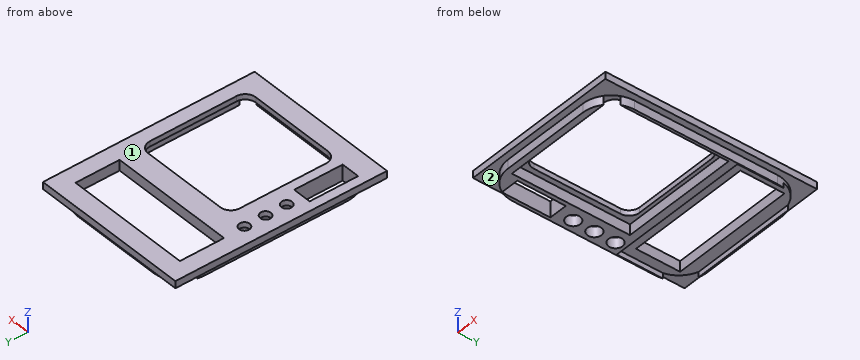
Autodesk Fusion 360 part; units mm, degrees
sketch "Skizze1" plane through (0, 0, 0) normal (0, 0, 1) x (1, 0, 0)
  line L0 (-52.263, 59.6389) -> (37.737, 59.6389)
  line L1 (37.737, 59.6389) -> (37.737, -60.3611)
  line L2 (37.737, -60.3611) -> (-52.263, -60.3611)
  line L3 (-52.263, -60.3611) -> (-52.263, 59.6389)
  dimension "d1" = 90
  dimension "d2" = 120
extrude "Extrusion1" add sketch "Skizze1" against normal blind 3
extrude "Extrusion2" add 1 faces at (-22.263, 19.6389, 0) along direction (0, 0, 1) blind 1
sketch "Skizze2" plane through (0, 0, 1) normal (0, 0, 1) x (-1, 0, 0)
  line L0 (52.263, 60.3611) -> (-37.737, 60.3611)
  line L1 (-37.737, 60.3611) -> (-37.737, -59.6389)
  line L2 (-37.737, -59.6389) -> (52.263, -59.6389)
  line L3 (52.263, -59.6389) -> (52.263, 60.3611)
  line L4 (25.263, -11.6389) -> (-23.737, -11.6389)
  line L5 (-29.737, -5.6389) -> (-29.737, 43.3611)
  line L6 (-23.737, 49.3611) -> (25.263, 49.3611)
  line L7 (31.263, 43.3611) -> (31.263, -5.6389)
  line L8 (33.263, -12.6389) -> (-31.737, -12.6389)
  line L9 (-31.737, -12.6389) -> (-31.737, 52.3611)
  line L10 (-31.737, 52.3611) -> (33.263, 52.3611)
  line L11 (33.263, 52.3611) -> (33.263, -12.6389)
  line L12 (42.763, -49.1389) -> (-28.237, -49.1389)
  line L13 (-28.237, -49.1389) -> (-28.237, -24.1389)
  line L14 (-28.237, -24.1389) -> (42.763, -24.1389)
  line L15 (42.763, -24.1389) -> (42.763, -49.1389)
  circle A0 centre (42.263, -12.1389) radius 3
  circle A1 centre (42.263, -0.1389) radius 3
  circle A2 centre (42.263, 11.8611) radius 3
  line L16 (47.013, 20.8611) -> (36.513, 20.8611)
  line L17 (36.513, 20.8611) -> (36.513, 48.3611)
  line L18 (36.513, 48.3611) -> (47.013, 48.3611)
  line L19 (47.013, 48.3611) -> (47.013, 20.8611)
  arc A3 (-29.737, -5.6389) -> (-23.737, -11.6389) centre (-23.737, -5.6389) ccw
  arc A4 (25.263, -11.6389) -> (31.263, -5.6389) centre (25.263, -5.6389) ccw
  arc A5 (31.263, 43.3611) -> (25.263, 49.3611) centre (25.263, 43.3611) ccw
  arc A6 (-23.737, 49.3611) -> (-29.737, 43.3611) centre (-23.737, 43.3611) ccw
  point P0 (31.263, -11.6389)
  point P1 (-29.737, -11.6389)
  point P2 (31.263, 49.3611)
  dimension "d7" = 61
  dimension "d8" = 61
  dimension "d10" = 11
  dimension "d11" = 65
  dimension "d12" = 65
  dimension "d13" = 8
  dimension "d19" = 25
  dimension "d20" = 71
  dimension "d23" = 8
  dimension "d24" = 6
  dimension "d25" = 6
  dimension "d26" = 9
  dimension "d28" = 6
  dimension "d29" = 6
  dimension "d30" = 12
  dimension "d31" = 9
  dimension "d32" = 9
  dimension "d33" = 12
  dimension "d34" = 10.5
  dimension "d35" = 27.5
  dimension "d36" = 12
  dimension "d37" = 5.25
  dimension "d62" = 6
  dimension "d63" = 6
  dimension "d82" = 12
sketch "Skizze3" plane through (0, 0, -3) normal (0, 0, -1) x (1, 0, 0)
  line L0 (37.737, 60.3611) -> (-52.263, 60.3611)
  line L1 (-52.263, 60.3611) -> (-52.263, -59.6389)
  line L2 (-52.263, -59.6389) -> (37.737, -59.6389)
  line L3 (37.737, -59.6389) -> (37.737, 60.3611)
  line L4 (-32.763, 56.8611) -> (18.237, 56.8611)
  line L5 (34.237, 40.8611) -> (34.237, -56.1389)
  line L6 (34.237, -56.1389) -> (-48.763, -56.1389)
  line L7 (-48.763, -56.1389) -> (-48.763, 40.8611)
  arc A0 (34.237, 40.8611) -> (18.237, 56.8611) centre (18.237, 40.8611) ccw
  arc A1 (-32.763, 56.8611) -> (-48.763, 40.8611) centre (-32.763, 40.8611) ccw
  line L8 (-52.263, 0.3611) -> (37.737, 0.3611)
  arc A2 (-48.763, -40.1389) -> (-32.763, -56.1389) centre (-32.763, -40.1389) ccw
  arc A3 (18.237, -56.1389) -> (34.237, -40.1389) centre (18.237, -40.1389) ccw
  dimension "d38" = 3.5
  dimension "d39" = 3.5
  dimension "d40" = 3.5
  dimension "d41" = 3.5
  dimension "d45" = 16
  dimension "d46" = 16
extrude "Extrusion3" add sketch "Skizze3" along normal blind 5 contours L4 L5 L7 A0 A1 L8 | L5 L6 L7 L8 A2 A3
extrude "Extrusion4" cut sketch "Skizze2" against normal blind 9 contours A1
extrude "Extrusion5" cut sketch "Skizze2" against normal blind 9 contours A0 | A2
sketch "Skizze4" plane through (0, 0, -8) normal (0, 0, -1) x (1, 0, 0)
  circle A0 centre (-42.263, -12.1389) radius 3
  circle A1 centre (-42.263, 11.8611) radius 3
  circle A2 centre (-42.263, -0.1389) radius 3
  arc A3 (-48.763, -40.1389) -> (-32.763, -56.1389) centre (-32.763, -40.1389) ccw
  line L0 (-32.763, -56.1389) -> (18.237, -56.1389)
  arc A4 (18.237, -56.1389) -> (34.237, -40.1389) centre (18.237, -40.1389) ccw
  line L1 (34.237, -40.1389) -> (34.237, 40.8611)
  arc A5 (34.237, 40.8611) -> (18.237, 56.8611) centre (18.237, 40.8611) ccw
  line L2 (18.237, 56.8611) -> (-32.763, 56.8611)
  arc A6 (-32.763, 56.8611) -> (-48.763, 40.8611) centre (-32.763, 40.8611) ccw
  line L3 (-48.763, 40.8611) -> (-48.763, -40.1389)
  circle A7 centre (-42.263, 11.8611) radius 4
  circle A8 centre (-42.263, -0.1389) radius 4
  circle A9 centre (-42.263, -12.1389) radius 4
  dimension "d53" = 8
  dimension "d54" = 8
  dimension "d55" = 8
extrude "Extrusion6" cut sketch "Skizze4" against normal blind 6 contours A7 | A8 | A9
extrude "Extrusion7" cut sketch "Skizze2" against normal blind 9 contours L16 L17 L18 L19
extrude "Extrusion8" cut sketch "Skizze2" against normal blind 9 contours L12 L13 L14 L15
extrude "Extrusion9" cut sketch "Skizze2" against normal blind 9 contours L4 L5 L6 L7 A3 A4 A5 A6
sketch "Skizze5" plane through (0, 0, -8) normal (0, 0, -1) x (1, 0, 0)
  line L0 (-25.263, 49.3611) -> (23.737, 49.3611)
  arc A0 (29.737, 43.3611) -> (23.737, 49.3611) centre (23.737, 43.3611) ccw
  line L1 (29.737, 43.3611) -> (29.737, -5.6389)
  arc A1 (23.737, -11.6389) -> (29.737, -5.6389) centre (23.737, -5.6389) ccw
  line L2 (23.737, -11.6389) -> (-25.263, -11.6389)
  arc A2 (-31.263, -5.6389) -> (-25.263, -11.6389) centre (-25.263, -5.6389) ccw
  line L3 (-31.263, -5.6389) -> (-31.263, 43.3611)
  arc A3 (-25.263, 49.3611) -> (-31.263, 43.3611) centre (-25.263, 43.3611) ccw
  line L4 (28.237, -24.1389) -> (28.237, -49.1389)
  line L5 (28.237, -49.1389) -> (-42.763, -49.1389)
  line L6 (-42.763, -49.1389) -> (-42.763, -24.1389)
  line L7 (-42.763, -24.1389) -> (28.237, -24.1389)
  line L8 (-47.013, 20.8611) -> (-47.013, 48.1369)
  arc A4 (-47.013, 48.1369) -> (-48.763, 40.8611) centre (-32.763, 40.8611) ccw
  line L9 (-48.763, 40.8611) -> (-48.763, -40.1389)
  arc A5 (-48.763, -40.1389) -> (-32.763, -56.1389) centre (-32.763, -40.1389) ccw
  line L10 (-32.763, -56.1389) -> (18.237, -56.1389)
  arc A6 (18.237, -56.1389) -> (34.237, -40.1389) centre (18.237, -40.1389) ccw
  line L11 (34.237, -40.1389) -> (34.237, 40.8611)
  arc A7 (34.237, 40.8611) -> (18.237, 56.8611) centre (18.237, 40.8611) ccw
  line L12 (18.237, 56.8611) -> (-32.763, 56.8611)
  arc A8 (-32.763, 56.8611) -> (-46.8963, 48.3611) centre (-32.763, 40.8611) ccw
  line L13 (-46.8963, 48.3611) -> (-36.513, 48.3611)
  line L14 (-36.513, 48.3611) -> (-36.513, 20.8611)
  line L15 (-36.513, 20.8611) -> (-47.013, 20.8611)
  circle A9 centre (-42.263, 11.8611) radius 4
  circle A10 centre (-42.263, -0.1389) radius 4
  circle A11 centre (-42.263, -12.1389) radius 4
  line L16 (32.737, -13.6389) -> (-34.263, -13.6389)
  line L17 (-34.263, -13.6389) -> (-34.263, 53.3611)
  line L18 (-34.263, 53.3611) -> (32.737, 53.3611)
  line L19 (32.737, 53.3611) -> (32.737, -13.6389)
  line L20 (37.737, 60.3611) -> (37.737, -59.6389)
  line L21 (-52.263, 60.3611) -> (37.737, 60.3611)
  dimension "d66" = 67
  dimension "d67" = 67
  dimension "d68" = 5
  dimension "d69" = 7
extrude "Extrusion10" cut sketch "Skizze5" against normal blind 6 contours A7 L16 L17 L18 L19
sketch "Skizze6" plane through (0, 0, 1) normal (0, 0, 1) x (-1, 0, 0)
  line L0 (42.763, -49.1389) -> (-28.237, -49.1389)
  line L1 (-28.237, -49.1389) -> (-28.237, -24.1389)
sketch "Skizze7" plane through (0, 0, -8) normal (0, 0, -1) x (1, 0, 0)
  line L0 (-34.263, 53.3611) -> (28.2245, 53.3611)
  arc A0 (28.2245, 53.3611) -> (18.237, 56.8611) centre (18.237, 40.8611) ccw
  line L1 (18.237, 56.8611) -> (-32.763, 56.8611)
  arc A1 (-32.763, 56.8611) -> (-46.8963, 48.3611) centre (-32.763, 40.8611) ccw
  line L2 (-46.8963, 48.3611) -> (-36.513, 48.3611)
  line L3 (-36.513, 48.3611) -> (-36.513, 20.8611)
  line L4 (-36.513, 20.8611) -> (-47.013, 20.8611)
  line L5 (-47.013, 20.8611) -> (-47.013, 48.1369)
  arc A2 (-47.013, 48.1369) -> (-48.763, 40.8611) centre (-32.763, 40.8611) ccw
  line L6 (-48.763, 40.8611) -> (-48.763, -40.1389)
  arc A3 (-48.763, -40.1389) -> (-32.763, -56.1389) centre (-32.763, -40.1389) ccw
  line L7 (-32.763, -56.1389) -> (18.237, -56.1389)
  arc A4 (18.237, -56.1389) -> (34.237, -40.1389) centre (18.237, -40.1389) ccw
  line L8 (34.237, -40.1389) -> (34.237, 40.8611)
  arc A5 (34.237, 40.8611) -> (32.737, 47.625) centre (18.237, 40.8611) ccw
  line L9 (32.737, 47.625) -> (32.737, -13.6389)
  line L10 (32.737, -13.6389) -> (-34.263, -13.6389)
  line L11 (-34.263, -13.6389) -> (-34.263, 53.3611)
  line L12 (28.237, -24.1389) -> (28.237, -49.1389)
  line L13 (28.237, -49.1389) -> (-42.763, -49.1389)
  line L14 (-42.763, -49.1389) -> (-42.763, -24.1389)
  line L15 (-42.763, -24.1389) -> (28.237, -24.1389)
  circle A6 centre (-42.263, 11.8611) radius 4
  circle A7 centre (-42.263, -0.1389) radius 4
  circle A8 centre (-42.263, -12.1389) radius 4
  line L16 (33.737, -55.3889) -> (-48.263, -55.3889)
  line L17 (-48.263, -55.3889) -> (-48.263, -17.8889)
  line L18 (-48.263, -17.8889) -> (33.737, -17.8889)
  line L19 (33.737, -17.8889) -> (33.737, -55.3889)
  line L20 (-42.763, -49.1389) -> (28.237, -49.1389)
  line L21 (28.237, -49.1389) -> (28.237, -24.1389)
  dimension "d76" = 82
  dimension "d77" = 37.5
  dimension "d78" = 6.25
  dimension "d79" = 5.5
extrude "Extrusion11" cut sketch "Skizze7" against normal blind 3 contours A4 L16 L19 | A3 A4 L16 L17 L18 L19 | A3 L16 L17
The model under review builds one solid part; all positions refer to its coordinate system, in mm. Face numbers are marked on the shaded views. A direction names the side the tool comes from. Coordinates: 2 decimals unless noted, no trailing zeros. Write each loop counter-clockwise with the first axis right and the second up, starting at its lowest first coordinate (ties: lowest second). Pieces come first, ordered by that corner, then holes. Notation, with made-up numbers: (19.25, 12) -> (77.25, 12) arc R27 cw to (77.25, 40) -> close; hole circle Ø8 at (62, 81.25). An arc over 180 degrees is marked (long way). One line per item, written item: value. Start each with the question number.
Q1. Add section D-D, the plane z = -0.5. Give the boundary of the cut face in (x, y).
Q2. To check wall thickness, follow probe 1 along X at (y, z) = (-14.5, -5.5); probe 2 along Y at (x, z) = (14, -6); probe 3 along Y at (x, z) = (-2.5, 0.5). State the ranges of each line that lie inside material, in increasing order.
Q3. Clearance check with flat-ended pins moving along their axes: P1, Ø0.9, axis at y = 26.5, z = -6, coming from the +X side; P2, Ø1.8, axis at x = -10, z = -4, coming from the +Y side; P3, Ø2.5, axis at x = -6, z = -6.5, coming from the -Y side; P4, Ø6.5, axis at x = -42.26, y = 12.14, coming from the +Z side. State where each tip first meets the part, or that it passes through.
Q4. Add section B-B, the plane x = -12.5. Give the boundary of the cut face in (y, z).
Q5. Add section C-C, the plane y = 38. Give the boundary of the cut face in (x, z).
Q6. Add section A-A, the plane y = -30. Give the boundary of the cut face in (x, z), then the cut area to 3 significant figures.
Q7. For the marked faces 1 and 2, list the 3-axis set-ups (+Z, -Z, +X, -X, +Y, -Y) from which the entire face can be reached by the end or side of a thin tool; tool diameter is ignored.
Response:
1. outline: (-52.26, -60.36) -> (37.74, -60.36) -> (37.74, 59.64) -> (-52.26, 59.64) -> close; hole (-47.01, -48.36) -> (-36.51, -48.36) -> (-36.51, -20.86) -> (-47.01, -20.86) -> close; hole circle Ø6 at (-42.26, -11.86); hole circle Ø6 at (-42.26, 0.14); hole circle Ø6 at (-42.26, 12.14); hole (-42.76, 24.14) -> (28.24, 24.14) -> (28.24, 49.14) -> (-42.76, 49.14) -> close; hole (-31.26, -43.36) arc R6 ccw to (-25.26, -49.36) -> (23.74, -49.36) arc R6 ccw to (29.74, -43.36) -> (29.74, 5.64) arc R6 ccw to (23.74, 11.64) -> (-25.26, 11.64) arc R6 ccw to (-31.26, 5.64) -> close
2. probe 1: -48.76 to -45.27, -39.26 to -34.26, 32.74 to 34.24
2. probe 2: -56.86 to -53.36, 13.64 to 17.89, 55.39 to 56.14
2. probe 3: -60.36 to -49.36, 11.64 to 24.14, 49.14 to 59.64
3. P1: x = 34.24
3. P2: y = 56.14
3. P3: y = -56.86
3. P4: z = 1
4. outline: (-60.36, -3) -> (-56.86, -3) -> (-56.86, -8) -> (-53.36, -8) -> (-53.36, -2) -> (-49.36, -2) -> (-49.36, 1) -> (-60.36, 1) -> close; (11.64, -2) -> (13.64, -2) -> (13.64, -8) -> (17.89, -8) -> (17.89, -5) -> (24.14, -5) -> (24.14, 1) -> (11.64, 1) -> close; (49.14, -5) -> (55.39, -5) -> (55.39, -8) -> (56.14, -8) -> (56.14, -3) -> (59.64, -3) -> (59.64, 1) -> (49.14, 1) -> close
5. outline: (-52.26, -3) -> (-48.76, -3) -> (-48.76, -8) -> (-48.26, -8) -> (-48.26, -5) -> (-42.76, -5) -> (-42.76, 1) -> (-52.26, 1) -> close; (28.24, -5) -> (33.74, -5) -> (33.74, -8) -> (34.24, -8) -> (34.24, -3) -> (37.74, -3) -> (37.74, 1) -> (28.24, 1) -> close
6. outline: (-52.26, -3) -> (-48.76, -3) -> (-48.76, -8) -> (-47.01, -8) -> (-47.01, 1) -> (-52.26, 1) -> close; (-36.51, -8) -> (-34.26, -8) -> (-34.26, -2) -> (-31.26, -2) -> (-31.26, 1) -> (-36.51, 1) -> close; (29.74, -2) -> (32.74, -2) -> (32.74, -8) -> (34.24, -8) -> (34.24, -3) -> (37.74, -3) -> (37.74, 1) -> (29.74, 1) -> close
6. area: 95.5 mm²
7. face 1: +Z, +X, -X, +Y, -Y
7. face 2: -Z
